For this review, take the finished solid that the model builds, in its own axes (mm). Round coordinates to 2 decimals unless told otherwise and drop trailing zeros. Write each loop counter-clockwise with the first axis right and the second up, starting at its lowest first coordinate (ties: lowest second). Pieces come first, ordered by that corner, then holes. Notation, with made-up numbers: M -21,26 L -17,26 A15 ccw -17,38 Z; hole C 80,1.5 d11. An arc over 180 degrees is marked long. One line per question, with ' | ' between items.
Autodesk Inventor part; units mm, degrees
ref_plane "YZ Plane" through (0, 0, 0) normal (1, 0, 0) x (0, 1, 0)
ref_plane "XZ Plane" through (0, 0, 0) normal (0, 1, 0) x (-1, 0, 0)
ref_plane "XY Plane" through (0, 0, 0) normal (0, 0, 1) x (1, 0, 0)
sketch "Sketch1" plane through (0, 0, 0) normal (0, 0, 1) x (1, 0, 0)
  line L0 (-173.3804, -25.4) -> (173.3804, -25.4)
  line L1 (176.5554, -22.225) -> (176.5554, 22.225)
  line L2 (173.3804, 25.4) -> (-173.3804, 25.4)
  line L3 (-176.5554, 22.225) -> (-176.5554, -22.225)
  circle A0 centre (-159.0929, 0) radius 11.1125
  circle A1 centre (155.9179, 0) radius 14.2875
  arc A2 (-176.5554, -22.225) -> (-173.3804, -25.4) centre (-173.3804, -22.225) ccw
  arc A3 (173.3804, -25.4) -> (176.5554, -22.225) centre (173.3804, -22.225) ccw
  arc A4 (176.5554, 22.225) -> (173.3804, 25.4) centre (173.3804, 22.225) ccw
  arc A5 (-173.3804, 25.4) -> (-176.5554, 22.225) centre (-173.3804, 22.225) ccw
  point P0 (0, 0)
  point P1 (-176.5554, -25.4)
  point P2 (176.5554, 25.4)
  point P3 (176.5554, -25.4)
  point P4 (-176.5554, 25.4)
  point P5 (-176.5554, 0)
  point P6 (0, 25.4)
  dimension "d5" = 315.0108
  dimension "d6" = 22.225
  dimension "d7" = 20.6375
  dimension "d8" = 17.4625
  dimension "d9" = 50.8
  dimension "d11" = 3.175
  dimension "d16" = 28.575
extrude "Extrusion1" add sketch "Sketch1" along normal blind 25.4
sketch "Sketch2" plane through (0, 0, 0) normal (1, 0, 0) x (0, 1, 0)
  line L0 (25.4, 25.4) -> (22.225, 25.4)
  line L1 (-22.225, 25.4) -> (22.225, 25.4)
  line L2 (-22.225, 25.4) -> (-25.4, 25.4)
  line L3 (-25.4, 0) -> (-25.4, 25.4)
  line L4 (-22.225, 0) -> (-25.4, 0)
  line L5 (-22.225, 0) -> (22.225, 0)
  line L6 (25.4, 0) -> (22.225, 0)
  line L7 (25.4, 0) -> (25.4, 25.4)
  line L8 (23.8125, 23.8125) -> (6.35, 23.8125)
  line L9 (6.35, 23.8125) -> (-6.35, 23.8125)
  line L10 (-6.35, 23.8125) -> (-23.8125, 23.8125)
  line L11 (-23.8125, 23.8125) -> (-23.8125, 1.5875)
  line L12 (-23.8125, 1.5875) -> (-6.35, 1.5875)
  line L13 (-6.35, 1.5875) -> (6.35, 1.5875)
  line L14 (6.35, 1.5875) -> (23.8125, 1.5875)
  line L15 (23.8125, 1.5875) -> (23.8125, 23.8125)
  dimension "d15" = 1.5875
extrude "Extrusion2" cut sketch "Sketch2" along normal through all both and the other way through all contours L15 L14 L13 L12 L11 L10 L9 L8
properties part number "SideBar13v2" material "Aluminum 6061"
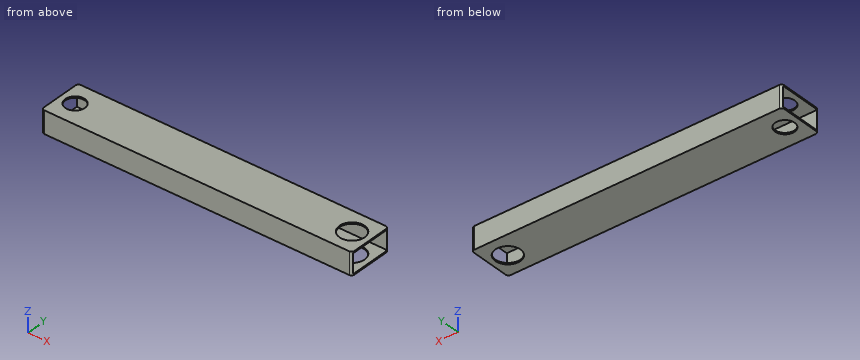
Item 1: Take a section at C-C (x = -106.5). Write out the cut boundary in (y, z).
Results:
outline: M -25.4,0 L 25.4,0 L 25.4,25.4 L -25.4,25.4 Z; hole M -23.81,1.59 L 23.81,1.59 L 23.81,23.81 L -23.81,23.81 Z
Item 2: To check wall thickness, follow line 1 along X through (y, z) = (0, 0.85); line 2 along Z through (x, y) = (13.5, -2.5); line 3 along Y through (x, z) = (94.5, 22). State the ranges of each line that lie inside material, in increasing order. Write a range as from..to.
Results:
line 1: -176.56..-170.21, -147.98..141.63, 170.21..176.56 | line 2: 0..1.59, 23.81..25.4 | line 3: -25.4..-23.81, 23.81..25.4
Item 3: Take a section at A-A (y = 0). Write out the cut boundary in (x, z), then the cut area to 3 significant figures.
Results:
outline: M -176.56,0 L -170.21,0 L -170.21,1.59 L -176.56,1.59 Z; M -176.56,23.81 L -170.21,23.81 L -170.21,25.4 L -176.56,25.4 Z; M -147.98,0 L 141.63,0 L 141.63,1.59 L -147.98,1.59 Z; M -147.98,23.81 L 141.63,23.81 L 141.63,25.4 L -147.98,25.4 Z; M 170.21,0 L 176.56,0 L 176.56,1.59 L 170.21,1.59 Z; M 170.21,23.81 L 176.56,23.81 L 176.56,25.4 L 170.21,25.4 Z | area: 960 mm2
